Can you work these out from the model? Positions are in its coordinate system, mm. Face numbers are marked on the shaded views. A direction names the side the tool comes from. Coordinates: 2 decimals unless noted, no trailing zeros. Order: outer loops, then holes, each group sorted by start corner. A loop starts at its lowest first (then second) coordinate and runs counter-clockwise, first axis right, second up. Notation, with made-up numbers: (62, -30) -> (95, -30) arc R27 cw to (95, -1) -> close; hole circle Ø9 at (65.25, -33.75). An arc over 180 degrees is marked (long way). Answer as CSV lines item,"result".
from build123d import *

# Parameters (mm, degrees)
BOSS_EXTRUDE1_DEPTH             = 22.7
SKETCH13_R                      = 5.9
BOSS_EXTRUDE2_DEPTH             = 4.6
TAP_DRILL_FOR_M3X0_5_TAP1_D     = 2.5
TAP_DRILL_FOR_M3X0_5_TAP1_DEPTH = 3
TAP_DRILL_FOR_M3X0_5_TAP1_TIP   = 0.751075774


with BuildPart() as part:
    # Sketch4 → Revolve1 (revolve)
    with BuildSketch(Plane(origin=(0, 0, 0), x_dir=(0, 0, -1), z_dir=(1, 0, 0))):
        Polygon((0, 0), (0, 18.5), (24.3, 18.5), (24.3, 17.5), (50, 17.5), (50, 0), align=None)
    revolve(axis=Axis((0, 0, 0), (0, 0, -1)))

    # Sketch12 → Boss-Extrude1 (add)
    with BuildSketch(Plane.XY):
        with BuildLine():
            Line((-1.658312395, -4.6), (1.658312395, -4.6))
            ThreePointArc((1.658312395, -4.6), (0, -10.1), (-1.658312395, -4.6))
        make_face()
    extrude(amount=BOSS_EXTRUDE1_DEPTH)

    # Sketch13 → Boss-Extrude2 (add)
    with BuildSketch(Plane.XY):
        with Locations((0, -7.1)):
            Circle(SKETCH13_R)
    extrude(amount=BOSS_EXTRUDE2_DEPTH)

    # Tap Drill for M3x0.5 Tap1
    with Locations(Plane.XY):
        with Locations((15.5, 0), (-15.5, 0), (-7.75, 13.423393759), (-7.75, -13.423393759)):
            Hole(TAP_DRILL_FOR_M3X0_5_TAP1_D / 2, depth=TAP_DRILL_FOR_M3X0_5_TAP1_DEPTH)
            with Locations((0, 0, -(TAP_DRILL_FOR_M3X0_5_TAP1_DEPTH + TAP_DRILL_FOR_M3X0_5_TAP1_TIP / 2))):  # 118° drill point
                Cone(0, TAP_DRILL_FOR_M3X0_5_TAP1_D / 2, TAP_DRILL_FOR_M3X0_5_TAP1_TIP, mode=Mode.SUBTRACT)


solid = part.part
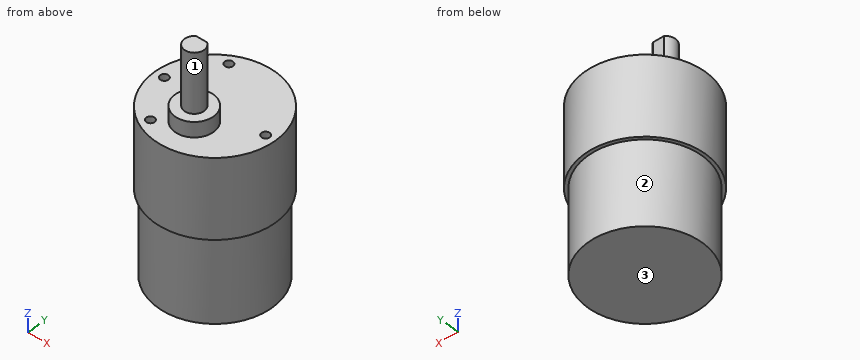
Q1. If I drill on line 1 (Y direction, x = -7.75, z = -1.1); line 2 (Z direction, x = -2, y = 5.5); line 3 (Z direction, x = -1.5, y = -4), over which ranges is the centre line in solid material (lowest first)?
Solution:
line 1,"-16.8 to -14.67, -12.17 to 12.17, 14.67 to 16.8"
line 2,"-50 to 0"
line 3,"-50 to 4.6"
Q2. Imagine slicing it at A-A (x = 0). List the corners of the cut face in (y, z) for me.
Solution:
outline,"(-18.5, -24.3) -> (-17.5, -24.3) -> (-17.5, -50) -> (17.5, -50) -> (17.5, -24.3) -> (18.5, -24.3) -> (18.5, 0) -> (-1.2, 0) -> (-1.2, 4.6) -> (-4.6, 4.6) -> (-4.6, 22.7) -> (-10.1, 22.7) -> (-10.1, 4.6) -> (-13, 4.6) -> (-13, 0) -> (-18.5, 0) -> close"
Q3. Imagine slicing it at C-C (z = 10.5). List the corners of the cut face in (x, y) for me.
Solution:
outline,"(-1.66, -4.6) arc R3 ccw (long way) to (1.66, -4.6) -> close"
Q4. Imagine slicing it at D-D (x = 5). List the corners of the cut face in (y, z) for me.
Solution:
outline,"(-17.81, -24.3) -> (-16.77, -24.3) -> (-16.77, -50) -> (16.77, -50) -> (16.77, -24.3) -> (17.81, -24.3) -> (17.81, 0) -> (-3.97, 0) -> (-3.97, 4.6) -> (-10.23, 4.6) -> (-10.23, 0) -> (-17.81, 0) -> close"
Q5. Which directions (+Z, -Z, +X, -X, +Y, -Y) give clear straight access to the entire face, cutting with the end or side of a thin tool? Please do the marked faces 1, 2 and 3.
Solution:
face 1,"+Z"
face 2,"-Z"
face 3,"-Z, +X, -X, +Y, -Y"
Q6. For P1, Ø10, axis at x = 6.5, y = 11, coming from the +Z side; P2, Ø2, axis at x = -7.75, y = 13.42, coming from the +Z side; P3, Ø1.5, axis at x = -1, y = -10, coming from the +Z side; P4, Ø5, axis at y = -3.5, z = 11.5, coming from the -X side, each with a flat end and sliding along its axis, tell me the tip position at first contact or that it passes through.
Solution:
P1,"z = 0"
P2,"z = -3.15"
P3,"z = 22.7"
P4,"x = -2.79"
Q7. Imagine slicing it at B-B (y = -7.1). List the corners of the cut face in (x, z) for me (3 decimals).
Solution:
outline,"(-17.083, -24.3) -> (-15.995, -24.3) -> (-15.995, -50) -> (15.995, -50) -> (15.995, -24.3) -> (17.083, -24.3) -> (17.083, 0) -> (5.9, 0) -> (5.9, 4.6) -> (3, 4.6) -> (3, 22.7) -> (-3, 22.7) -> (-3, 4.6) -> (-5.9, 4.6) -> (-5.9, 0) -> (-17.083, 0) -> close"
